from build123d import *

# Parameters (mm, degrees)
F0_W     = 131.0434639454
F0_H     = 157.073289156
F1_DEPTH = 38.1
F3_DEPTH = 25.4
F4_DEPTH = 31.75
F5_DEPTH = 25.4
F6_DEPTH = 25.4


with BuildPart() as f1:
    # F0 (on Front) → F1 (new body, symmetric)
    with BuildSketch(Plane.XZ):
        with Locations((0.093087554, -0.1957640052)):
            Rectangle(F0_W, F0_H)
    extrude(amount=F1_DEPTH, both=True)

    # F2 (on face) → F3 (join)
    with BuildSketch(Plane.XZ.offset(38.1)):
        Polygon((65.6148195267, -78.7324085832), (0.093087554, -0.1957640052), (0.0465768162, -0.2515134058), (0.093087554, -78.7324085832), align=None)
        Polygon((0.0464857272, -0.0978123848), (0, 78.3408805728), (-65.4286444187, 78.3408805728), (0.0113244291, -0.0977598578), align=None)
    extrude(amount=F3_DEPTH)

    # F4 (add): a face of the model
    f4_faces = [f1.faces().sort_by_distance(p)[0] for p in [
        (0.0930765329, -38.1, -0.1771720733),
    ]]
    extrude(f4_faces, amount=F4_DEPTH)

    # F5 (add): a face of the model
    f5_faces = [f1.faces().sort_by_distance(p)[0] for p in [
        (0.093087554, 38.1, -0.1957640052),
    ]]
    extrude(f5_faces, amount=-F5_DEPTH)

    # F6 (add): a face of the model
    f6_faces = [f1.faces().sort_by_distance(p)[0] for p in [
        (0.093087554, 38.1, -0.1957640052),
    ]]
    extrude(f6_faces, amount=-F6_DEPTH)


solid = f1.part
Design review of the part built by this model. Coordinates are the model's own, in mm. A direction names the side the tool comes from. Coordinates: 2 decimals unless noted, no trailing zeros. Order: outer loops, then holes, each group sorted by start corner. A loop starts at its lowest first (then second) coordinate and runs counter-clockwise, first axis right, second up. Notation, with made-up numbers: (-19.75, 18) -> (0.25, 18) arc R19 cw to (0.25, 26) -> close; hole circle Ø8 at (12, -7.75). An arc over 180 degrees is marked (long way). Use one line per item in the form item = value. Start each with the question number.
(1) Add section C-C on z = 69. State the section outline as (x, y) points.
(2) For faces 4 (the flat face through (-33.167, -66.631, 39.671)), 5 (the flat face through (25, -63.5, -48)), 6 (the flat face through (-65.429, -15, -1)), list the 3-axis set-ups (+Z, -Z, +X, -X, +Y, -Y) from which the entire face can be reached by the end or side of a thin tool; tool diameter is ignored.
(3) For probe 1 along Y at (x, z) = (-9, 12), list the stretches that pass through material, from the lowest coordinate up.
(4) The part is to be moulded in two halves that separate along Z. For faces 1 (the flat face through (-1, 38.1, 1)), 2 (the flat face through (-1, -15, -78.732)), 3 (the flat face through (-1, -15, 78.341)), say which applies: +Z half, -Z half, draft (parallel to the pull), parting line (faces both ways), or undercut.
(5) Add section A-A on z = -58.5. State the section outline as (x, y) points.
(6) Add section D-D on x = -27.5. State the section outline as (y, z) points.
(7) Add section B-B on x = 31.5. State the section outline as (y, z) points.
(8) Insertion check: pin 1 (8 mm diameter, centred on x = 13, z = -35, fed in from -Y). The pin has a flat end and moves straight along its axis. Give the tip position at first contact, or say it passes through.
Answer block:
q1.outline = (-65.43, -69.85) -> (-57.64, -69.85) -> (-57.64, -63.5) -> (0.01, -63.5) -> (0.01, -69.85) -> (65.61, -69.85) -> (65.61, 38.1) -> (-65.43, 38.1) -> close
q2.face_4 = +Z, -Y
q2.face_5 = -Z, -Y
q2.face_6 = +Z, -Z, -X, +Y, -Y
q3.probe_1 = -63.5 to 38.1
q4.face_1 = draft
q4.face_2 = -Z half
q4.face_3 = +Z half
q5.outline = (-65.43, -69.85) -> (0.08, -69.85) -> (0.08, -63.5) -> (48.74, -63.5) -> (48.74, -69.85) -> (65.61, -69.85) -> (65.61, 38.1) -> (-65.43, 38.1) -> close
q6.outline = (-69.85, -78.73) -> (38.1, -78.73) -> (38.1, 78.34) -> (-63.5, 78.34) -> (-63.5, 32.88) -> (-69.85, 32.88) -> close
q7.outline = (-69.85, -37.84) -> (-63.5, -37.84) -> (-63.5, -78.73) -> (38.1, -78.73) -> (38.1, 78.34) -> (-69.85, 78.34) -> close
q8.pin_1 = -63.5
